Geometry check sheet. Reference: the model listing, model coordinates, mm. Face numbers are marked on the shaded views. Coordinates: 2 decimals unless noted, no trailing zeros. Order: outer loops, then holes, each group sorted by start corner. A loop starts at its lowest first (then second) coordinate and runs counter-clockwise, first axis right, second up.
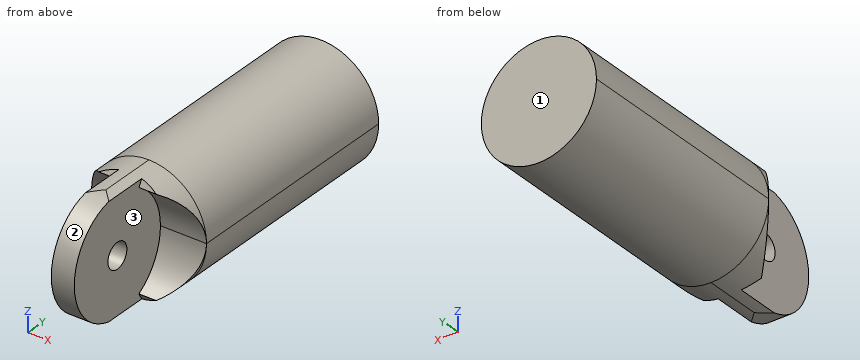
Autodesk Inventor part; units mm, degrees
ref_plane "YZ Plane" through (0, 0, 0) normal (1, 0, 0) x (0, 1, 0)
ref_plane "XZ Plane" through (0, 0, 0) normal (0, 1, 0) x (-1, 0, 0)
ref_plane "XY Plane" through (0, 0, 0) normal (0, 0, 1) x (1, 0, 0)
sketch "Sketch1" plane through (0, 0, 0) normal (0, 1, 0) x (-1, 0, 0)
  circle A0 centre (0, 0) radius 5
  dimension "d0" = 10
extrude "Extrusion1" add sketch "Sketch1" along normal blind 20
sketch "Sketch2" plane through (0, 0, 0) normal (1, 0, 0) x (0, 1, 0)
  circle A0 centre (-5, 0) radius 1.1
  line L0 (0, -5) -> (0, 5)
  circle A1 centre (-5, 0) radius 5
  line L1 (0, 5) -> (-5, 5)
  line L2 (-5, -5) -> (0, -5)
  line L3 (0, -5) -> (0, 5)
  point P0 (0, 0)
  dimension "d3" = 2.2
  dimension "d4" = 5
  dimension "d5" = 5
  dimension "d6" = 10
extrude "Extrusion2" add sketch "Sketch2" along normal mid plane 2
sketch "Sketch3" plane through (1, 0, 0) normal (1, 0, 0) x (0, 0, -1)
  circle A0 centre (0, -5) radius 1.1
  line L0 (0, -5) -> (4.3301, -2.5)
  line L1 (0, -5) -> (5, -5) construction
  line L2 (0, -5) -> (-4.3301, -2.5)
  line L3 (0, -5) -> (5, -5) construction
  circle A1 centre (0, -5) radius 1.1
  circle A2 centre (0, -5) radius 5
  line L4 (0, -5) -> (5, -2.1132)
  line L5 (0, -5) -> (-5, -2.1132)
  line L6 (-5, 0) -> (-5, -5)
  line L7 (-5, 0) -> (-5, -2.1132)
  line L8 (5, -2.1132) -> (5, 0)
  line L9 (5, 0) -> (-5, 0)
  line L10 (4.899, 0) -> (-4.899, 0)
  point P0 (0, 0)
  point P1 (0, 0)
  dimension "d9" = 5
  dimension "d10" = 30
  dimension "d11" = 5
  dimension "d12" = 150
  dimension "d13" = 2.1132
extrude "Extrusion3" add sketch "Sketch3" along normal blind 5 contours A2 L9 L8 L4 | L5 L6 L9 A2
mirror "Mirror1" about plane through (0, 0, 0) normal (1, 0, 0) of "Extrusion3"
sketch "Sketch4" plane through (0, 20, 0) normal (0, 1, 0) x (1, 0, 0)
  circle A0 centre (0, 0) radius 5
  circle A1 centre (0, 0) radius 10
  dimension "d16" = 10
  dimension "d17" = 20
extrude "Extrusion4" cut sketch "Sketch4" against normal through all
properties part number "Camera encase" material "Rubber"
Item 1: Sectioned sample at B-B (x = 0.5). Record the cut outline in (y, z), and give its area (3 significant figures).
Item 2: Sectioned sample at A-A (z = -4). Record the cut outline in (x, y).
Item 3: Thickness scan on line 1 along Z through (x, y) = (0.2, -5); line 2 along Z through (x, y) = (-2.5, 8.75); line 3 along X through (y, z) = (-7, 0.75). Record the ranges inside material, lowest first.
Item 4: Depth check by flat-ended pin: P1, Ø3, axis at y = 7.5, z = -0.5, coming from the +X side; P2, Ø5, axis at x = 4, z = -1.5, coming from the -Y side; P3, Ø3, axis at y = -6, z = -1.5, coming from the -X side. Enter the tip coordinate at first touch or a pass-through.
Item 5: Release check for a two-part mould opening along Z. For the marked faces 1, 2 and 3 record: pulls with the +Z half, pulls with the -Z half, needs draft (parallel to the pull), parting line crosses it, or undercut.
Item 6: Sectioned sample at C-C (y = 18.25). Record the cut outline in (x, z), and give its area (3 significant figures).
Item 7: Sectioned sample at D-D (z = -1.5). Record the cut outline in (x, y).
Geometry check:
1. outline: (-5.5, -4.97) - (20, -4.97) - (20, 4.97) - (-5.5, 4.97) arc R5 ccw to start; hole circle Ø2.2 at (-5, 0)
1. area: 284 mm2
2. outline: (-3, -2) - (-1, -2) - (-1, -8) - (1, -8) - (1, -2) - (3, -2) - (3, 20) - (-3, 20) - close
3. line 1: z = -5 to -1.1, 1.1 to 5
3. line 2: z = -4.33 to 4.33
3. line 3: x = -1 to 1
4. P1: stops at x = 5
4. P2: stops at y = -1.82
4. P3: stops at x = -1
5. face 1: needs draft
5. face 2: parting line crosses it
5. face 3: undercut
6. outline: circle Ø10 at (0, 0)
6. area: 78.5 mm2
7. outline: (-4.77, -0.23) - (-1, -0.23) - (-1, -9.77) - (1, -9.77) - (1, -0.23) - (4.77, -0.23) - (4.77, 20) - (-4.77, 20) - close
